Autodesk Inventor part; units mm, degrees
ref_plane "YZ Plane" through (0, 0, 0) normal (1, 0, 0) x (0, 1, 0)
ref_plane "XZ Plane" through (0, 0, 0) normal (0, 1, 0) x (-1, 0, 0)
ref_plane "XY Plane" through (0, 0, 0) normal (0, 0, 1) x (1, 0, 0)
sketch "Sketch1" plane through (0, 0, 0) normal (0, 0, 1) x (1, 0, 0)
  line L0 (0, 0) -> (0, 1910) construction
  line L1 (424.5155, 1910) -> (-415.4845, 1910)
  line L2 (-415.4845, 1910) -> (-1180, 1150)
  line L3 (-1180, 0) -> (-1180, 1150)
  line L4 (960, 0) -> (960, 1342.8524)
  line L5 (424.5155, 1910) -> (960, 1342.8524)
  circle A0 centre (0, 950) radius 265 construction
  line L6 (960, 0) -> (-1180, 0)
  circle A1 centre (-1701.6377, -269.2167) radius 188.5 construction
  circle A2 centre (-800, 80) radius 55.5
  circle A3 centre (0, 950) radius 170
  line L7 (0, 1215) -> (0, 1120) construction
  line L8 (-721.2646, 955) -> (721.2646, 955) construction
  line L9 (-169.9265, 955) -> (-174.9265, 955) construction
  line L10 (-174.9265, 960) -> (-174.9265, 950)
  line L11 (-174.9265, 960) -> (-169.7056, 960)
  line L12 (-174.9265, 950) -> (-170, 950)
  line L13 (169.9265, 955) -> (174.9265, 955) construction
  line L14 (174.9265, 960) -> (174.9265, 950)
  line L15 (169.7056, 960) -> (174.9265, 960)
  line L16 (174.9265, 950) -> (170, 950)
  line L17 (-174.9265, 970) -> (174.9265, 970)
  line L18 (174.9265, 970) -> (174.9265, 940)
  line L19 (174.9265, 940) -> (-174.9265, 940)
  line L20 (-174.9265, 940) -> (-174.9265, 970)
  arc A4 (-2.4999, 780.0184) -> (2.4999, 780.0184) centre (0, 780) ccw
  arc A5 (2.4999, 1119.9816) -> (-2.4999, 1119.9816) centre (0, 1120) ccw
  point P0 (0, 955)
  point P1 (-169.7056, 940)
  point P2 (169.7056, 940)
  point P3 (168.8194, 970)
  point P4 (-168.8194, 970)
  dimension "d52" = 530
  dimension "d72" = 340
  dimension "d1" = 840
  dimension "d3" = 1150
  dimension "d12" = 1180
  dimension "d13" = 950
  dimension "d14" = 111
  dimension "d15" = 1910
  dimension "d17" = -521.6377
  dimension "d18" = 377
  dimension "d19" = -269.2167
  dimension "d34" = 380
  dimension "d35" = 80
  dimension "d37" = 2140
  dimension "d53" = 5
  dimension "d54" = 10
  dimension "d55" = 30
  dimension "d67" = 5
  dimension "d68" = 5
  dimension "d69" = 780
  dimension "d71" = 1078
extrude "Extrusion1" add sketch "Sketch1" along normal blind 10 contours L5 L4 L6 L3 L2 L1 | A3 L19 L17 | L16 L18 L19 A3 | A3 L15 L14 L16 | A3 L17 L18 L15 | L19 L20 L12 A3 | A3 L11 L20 L17 | L12 L10 L11 A3
fillet "Fillet1" radius 10 4 edges at (-168.8194, 970, 5) (-169.7056, 940, 5) (168.8194, 970, 5) (169.7056, 940, 5)
sketch "Sketch4" plane through (0, 0, 0) normal (0, 0, 1) x (1, 0, 0)
  circle A0 centre (-51.6989, 1209.9081) radius 6.5
  arc A1 (-2.4999, 1119.9816) -> (-166.985, 981.875) centre (0, 950) ccw
  line L0 (0, 950) -> (0, 1196.7062) construction
  line L1 (-51.6989, 1209.9081) -> (0, 950) construction
  point P0 (0, 0)
  point P1 (-5, 1149.9375)
  dimension "d59" = 265
  dimension "d60" = 13
  dimension "d61" = 11.25
extrude "Extrusion4" cut sketch "Sketch4" along normal blind 10
pattern_circular "Circular Pattern3" count 16 over 360 about axis through (0, 950, 0) along (0, 0, 1) of "Extrusion4"
sketch "Sketch5" plane through (0, 0, 10) normal (0, 0, 1) x (1, 0, 0)
  circle A0 centre (51.6989, 1209.9081) radius 6.5
  circle A1 centre (147.2261, 1170.3394) radius 6.5
  circle A2 centre (220.3394, 1097.2261) radius 6.5
  circle A3 centre (259.9081, 1001.6989) radius 6.5
  circle A4 centre (259.9081, 898.3011) radius 6.5
  circle A5 centre (220.3394, 802.7739) radius 6.5
  circle A6 centre (147.2261, 729.6606) radius 6.5
  circle A7 centre (51.6989, 690.0919) radius 6.5
  circle A8 centre (-51.6989, 690.0919) radius 6.5
  circle A9 centre (-147.2261, 729.6606) radius 6.5
  circle A10 centre (-220.3394, 802.7739) radius 6.5
  circle A11 centre (-259.9081, 898.3011) radius 6.5
  circle A12 centre (-259.9081, 1001.6989) radius 6.5
  circle A13 centre (-220.3394, 1097.2261) radius 6.5
  circle A14 centre (-147.2261, 1170.3394) radius 6.5
  circle A15 centre (-51.6989, 1209.9081) radius 6.5
  line L0 (960, 1342.8524) -> (424.5155, 1910)
  line L1 (424.5155, 1910) -> (-415.4845, 1910)
  line L2 (-415.4845, 1910) -> (-1180, 1150)
  line L3 (-1180, 1150) -> (-1180, 0)
  line L4 (-1180, 0) -> (960, 0)
  line L5 (960, 0) -> (960, 1342.8524)
  arc A16 (2.4999, 780.0184) -> (168.6666, 928.75) centre (0, 950) ccw
  arc A17 (-2.4999, 780.0184) -> (2.4999, 780.0184) centre (0, 780) ccw
  arc A18 (-168.6666, 928.75) -> (-2.4999, 780.0184) centre (0, 950) ccw
  arc A19 (-158.7451, 940) -> (-168.6666, 928.75) centre (-158.7451, 930) ccw
  line L6 (-158.7451, 940) -> (158.7451, 940)
  arc A20 (168.6666, 928.75) -> (158.7451, 940) centre (158.7451, 930) ccw
  circle A21 centre (-800, 80) radius 55.5
  line L7 (157.1623, 970) -> (-157.1623, 970)
  arc A22 (-166.985, 981.875) -> (-157.1623, 970) centre (-157.1623, 980) ccw
  arc A23 (-2.4999, 1119.9816) -> (-166.985, 981.875) centre (0, 950) ccw
  arc A24 (2.4999, 1119.9816) -> (-2.4999, 1119.9816) centre (0, 1120) ccw
  arc A25 (166.985, 981.875) -> (2.4999, 1119.9816) centre (0, 950) ccw
  arc A26 (157.1623, 970) -> (166.985, 981.875) centre (157.1623, 980) ccw
  line L8 (424.5155, 1910) -> (-415.4845, 1910)
  line L9 (-380, 1910) -> (-380, 0)
  point P0 (0, 0)
  dimension "d73" = 1340
extrude "Extrusion5" cut sketch "Sketch5" against normal through all contours L5 L4 L9 L1 L0
properties part number "ДМФ 011 Стенка Корма ЛЕВ"
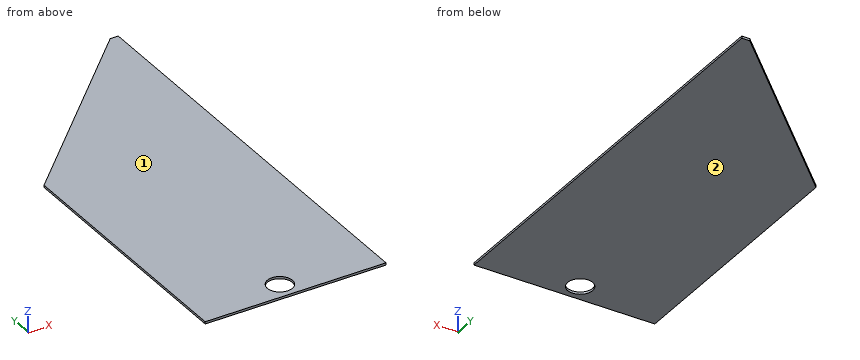
Geometry: final body of the model. Coordinates: model frame, mm. Face numbers are marked on the shaded views. Round coordinates to 2 decimals unless told otherwise and drop trailing zeros. Order: outer loops, then holes, each group sorted by start corner. A loop starts at its lowest first (then second) coordinate and runs counter-clockwise, first axis right, second up. Notation, with made-up numbers: (85.25, 13) - (129.25, 13) arc R17 cw to (129.25, 36) - close; hole circle Ø2 at (27.5, 10). An arc over 180 degrees is marked (long way). Write each question's results on one line, items separated by ' | '.
Item 1: Section C-C, the plane z = 5. Return the cut outline in (x, y).
Completed:
outline: (-1180, 0) - (-380, 0) - (-380, 1910) - (-415.48, 1910) - (-1180, 1150) - close; hole circle Ø111 at (-800, 80)
Item 2: Mould query, pull axis Z, two halves, no side actions, for the marked faces 1 and 2. Classes: pulls with the +Z half, pulls with the -Z half, needs draft (parallel to the pull), parting line crosses it, or undercut.
Completed:
face 1: pulls with the +Z half | face 2: pulls with the -Z half
Item 3: First-contact query: pin 1 Ø4 at (x, z) = (-467, 1.5) entering from +Y; pin 2 Ø5 at (x, z) = (-1072.5, 3) entering from +Y; pin 3 Ø2 at (y, z) = (1384, 6) entering from -X. Flat tips, straight axial feed; report the tip coordinate or a pass-through.
Completed:
pin 1: y = 1860.78 | pin 2: y = 1259.35 | pin 3: x = -945.62
Item 4: Section D-D, the plane x = -619.5. Return the cut outline in (y, z).
Completed:
outline: (0, 0) - (1707.19, 0) - (1707.19, 10) - (0, 10) - close
Item 5: Section B-B, the plane x = -800. Return the cut outline in (y, z), and give its area (3 significant figures).
Completed:
outline: (0, 0) - (24.5, 0) - (24.5, 10) - (0, 10) - close; (135.5, 0) - (1527.76, 0) - (1527.76, 10) - (135.5, 10) - close | area: 14,200 mm^2
Item 6: Section A-A, the plane y = 80. Return the cut outline in (x, z), and give its area (3 significant figures).
Completed:
outline: (-1180, 0) - (-855.5, 0) - (-855.5, 10) - (-1180, 10) - close; (-744.5, 0) - (-380, 0) - (-380, 10) - (-744.5, 10) - close | area: 6,890 mm^2
Item 7: Material intervals for line 1 along Y through (x, z) = (-778, 7); line 2 along Y through (x, z) = (-800, 8); line 3 along X through (y, z) = (101.5, 4.75), sorted ascending. Write a range as [from, to].
Completed:
line 1: [0, 29.05], [130.95, 1549.63] | line 2: [0, 24.5], [135.5, 1527.76] | line 3: [-1180, -851.17], [-748.83, -380]
